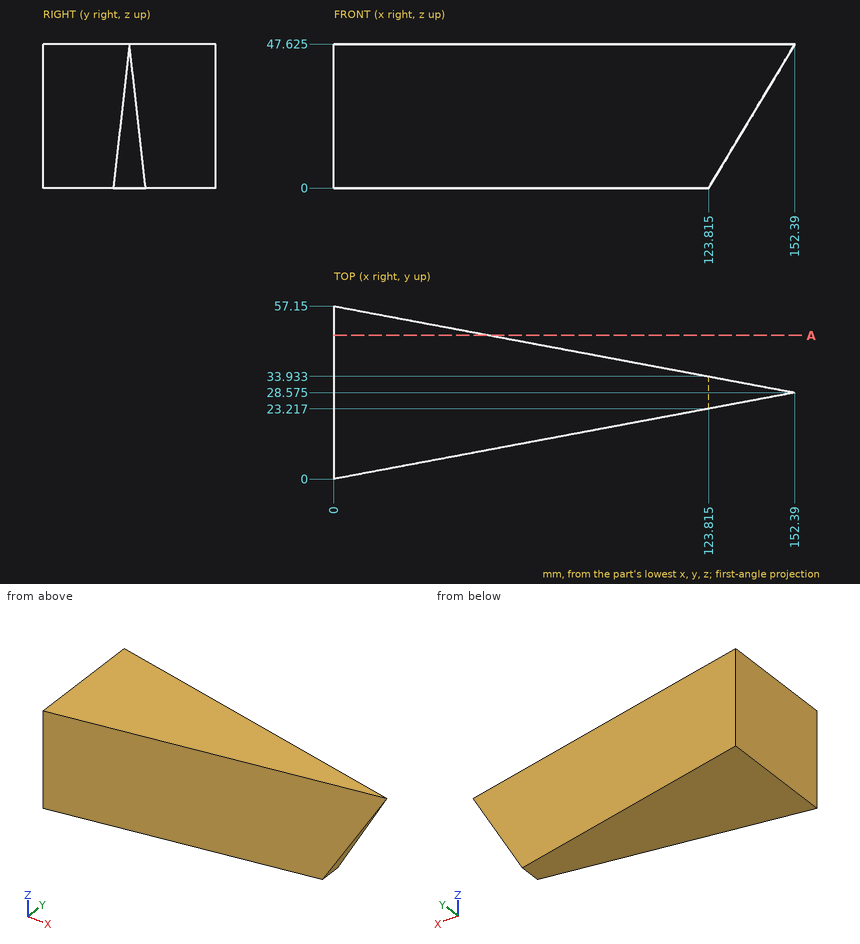
Can you work these out from the drawing? Everything is in mm from the part's minimum corner. Round coordinates to 2 decimals unless told otherwise and drop trailing zeros. Order: outer loops, then holes, each group sorted by start corner. A loop starts at its lowest first (then second) coordinate and runs counter-clockwise, first axis right, second up. Notation, with made-up numbers: (48, 32.5) - (83, 32.5) arc R31 ccw to (83, 60.5) - close; hole circle Ø10 at (12, -26). An arc over 180 degrees is marked (long way). Answer in a Markdown table with one row per item.
(1) For P1, Ø6, axis at x = 34.5, z = 28.5, coming from the -Y side; P2, Ø6, axis at x = 76, z = 40, coming from the -Y side; P3, Ø1, axis at x = 111.5, z = 41, coming from the +Y side, each with a flat end and sliding along its axis, tell me the tip position at first contact or that it passes through.
From the geometry:
| item | result |
|---|---|
| P1 | stops at y = 5.91 |
| P2 | stops at y = 13.69 |
| P3 | stops at y = 36.34 |
(2) Please list where these lines run through material, in increasing order: L1, parallel to Y at x = 90, z = 27 (1 decimal); L2, parallel to Y at x = 29.5, z = 38; L3, parallel to X at y = 27, z = 18.5 (1 decimal). Write a range as from..to.
From the geometry:
| item | result |
|---|---|
| L1 | y = 16.9..40.3 |
| L2 | y = 5.53..51.62 |
| L3 | x = 0..134.9 |
(3) Suppose I cut it at A-A, the plane y = 47.5. Please give me the cut outline in (x, z) (1 decimal), plus the area to 3 significant figures.
From the geometry:
| item | result |
|---|---|
| outline | (0, 0) - (51.5, 0) - (51.5, 47.6) - (0, 47.6) - close |
| area | 2,450 mm2 |
